```python
from build123d import *

# Parameters (mm, degrees)
SKETCH2_R           = 17.5
SKETCH2_R_2         = 2
BOSS_EXTRUDE1_DEPTH = 5
SKETCH3_R           = 10
BOSS_EXTRUDE2_DEPTH = 15


with BuildPart() as part:
    # Sketch2 → Boss-Extrude1 (new body)
    with BuildSketch(Plane(origin=(0, 0, 0), x_dir=(1, 0, 0), z_dir=(0, 1, 0))):
        with Locations(Location((0, 0, 0), (0, 0, 270))):
            Circle(SKETCH2_R)
        with Locations(Location((0, 13.75, 0), (0, 0, 270))):
            Circle(SKETCH2_R_2, mode=Mode.SUBTRACT)
        with Locations(Location((11.907849302, 6.875, 0), (0, 0, 270))):
            Circle(SKETCH2_R_2, mode=Mode.SUBTRACT)
        with Locations(Location((11.907849302, -6.875, 0), (0, 0, 270))):
            Circle(SKETCH2_R_2, mode=Mode.SUBTRACT)
        with Locations(Location((0, -13.75, 0), (0, 0, 270))):
            Circle(SKETCH2_R_2, mode=Mode.SUBTRACT)
        with Locations(Location((-11.907849302, -6.875, 0), (0, 0, 270))):
            Circle(SKETCH2_R_2, mode=Mode.SUBTRACT)
        with Locations(Location((-11.907849302, 6.875, 0), (0, 0, 270))):
            Circle(SKETCH2_R_2, mode=Mode.SUBTRACT)
    extrude(amount=BOSS_EXTRUDE1_DEPTH)

    # Sketch3 → Boss-Extrude2 (add)
    with BuildSketch(Plane(origin=(0, 5, 0), x_dir=(1, 0, 0), z_dir=(0, 1, 0))):
        with Locations(Location((0, 0, 0), (0, 0, 270))):
            Circle(SKETCH3_R)
    extrude(amount=BOSS_EXTRUDE2_DEPTH)


solid = part.part
```
Work out the finished part from the listing and answer in its coordinate system (mm). A direction names the side the tool comes from. Give positions to 0.01 mm unless a question says otherwise; leave off trailing zeros. Write each loop counter-clockwise with the first axis right and the second up, starting at its lowest first coordinate (ties: lowest second). Pieces come first, ordered by that corner, then holes. Notation, with made-up numbers: (-32.5, 88) -> (-21.5, 88) arc R16 ccw to (-21.5, 106) -> close; hole circle Ø6 at (44, 5). An arc over 180 degrees is marked (long way). Write item = value, one per line.
Q1. Section A-A on x = 0 is taken. Determine the outline of the cut face in (y, z), and give its area (3 significant figures).
Computed values:
outline = (0, -17.5) -> (5, -17.5) -> (5, -15.75) -> (0, -15.75) -> close; (0, -11.75) -> (5, -11.75) -> (5, -10) -> (20, -10) -> (20, 10) -> (5, 10) -> (5, 11.75) -> (0, 11.75) -> close; (0, 15.75) -> (5, 15.75) -> (5, 17.5) -> (0, 17.5) -> close
area = 435 mm^2
Q2. Flat-ended cylindrical pins translate along their axes: pin 1 Ø12 at (y, z) = (7, 7) entering from -X; pin 2 Ø3.5 at (x, z) = (0, 13.75) entering from -Y; pin 3 Ø3 at (x, z) = (-11.5, 6) entering from +Y; pin 4 Ø8 at (y, z) = (3, 7.5) entering from -X. Find the tip coordinate at first contact, or state that the pin passes through.
Computed values:
pin_1 = -17.45
pin_2 = through
pin_3 = 5
pin_4 = -17.15
Q3. Section D-D on y = 15.5 is taken. Determine the outline of the cut face in (x, z).
Computed values:
outline = circle Ø20 at (0, 0)
Q4. Section B-B on z = -14.5 is taken. Determine the outline of the cut face in (x, y), and give its area (3 significant figures).
Computed values:
outline = (-9.8, 0) -> (-1.85, 0) -> (-1.85, 5) -> (-9.8, 5) -> close; (1.85, 0) -> (9.8, 0) -> (9.8, 5) -> (1.85, 5) -> close
area = 79.4 mm^2
Q5. For a pull along X with two mould halves and no side action, classify faces 1 (the cylindrical face through (-13.125, 2.465, -8.462)), 2 (the flat face through (0, 0, 0)), 3 (the cylindrical face through (-9.76, 12.4, -2.17)) as pulls with the +X half, pulls with the -X half, needs draft (parallel to the pull), parting line crosses it, or undercut.
Computed values:
face_1 = undercut
face_2 = needs draft
face_3 = parting line crosses it
Q6. Section C-C on z = 8 is taken. Determine the outline of the cut face in (x, y), and give its area (3 significant figures).
Computed values:
outline = (-15.56, 0) -> (-13.56, 0) -> (-13.56, 5) -> (-15.56, 5) -> close; (-10.25, 0) -> (10.25, 0) -> (10.25, 5) -> (6, 5) -> (6, 20) -> (-6, 20) -> (-6, 5) -> (-10.25, 5) -> close; (13.56, 0) -> (15.56, 0) -> (15.56, 5) -> (13.56, 5) -> close
area = 303 mm^2
Q7. Consider line 1 along Y through (x, z) = (-11, 11.5); line 2 along X through (y, z) = (3.15, 13.75); line 3 along X through (y, z) = (1.75, -15). Determine where each line is inside the solid, lowest interval first.
Computed values:
line_1 = 0 to 5
line_2 = -10.83 to -2, 2 to 10.83
line_3 = -9.01 to -1.56, 1.56 to 9.01
Q8. A tool of negligible diameter and unlimited length cuts with its end or side. For faces 4 (the cylindrical face through (10.69, 2.46, -8.46)), 5 (the flat face through (-8, 5, 8)), from which of +Z, -Z, +X, -X, +Y, -Y can it reach the whole face along a straight path? Write none if from no direction.
Computed values:
face_4 = +Y, -Y
face_5 = +Y
